from build123d import *

# Parameters (mm, degrees)
SKETCH1_W                   = 42.3
SKETCH1_H                   = 46
SKETCH1_R                   = 12
SKETCH1_R_2                 = 1.7
BOSS_EXTRUDE1_DEPTH         = 2
BOSS_EXTRUDE4_DEPTH         = 2
BOSS_EXTRUDE6_REACH         = 76.681
SKETCH6_W                   = 2
SKETCH6_H                   = 39
M3_TAPPED_HOLE2_D           = 2.5
M3_TAPPED_HOLE2_CSINK_D     = 3.05
M3_TAPPED_HOLE2_CSINK_ANGLE = 90


with BuildPart() as part:
    # Sketch1 → Boss-Extrude1 (new body)
    with BuildSketch(Plane.XY):
        Rectangle(SKETCH1_W, SKETCH1_H)
        Circle(SKETCH1_R, mode=Mode.SUBTRACT)
        with Locations((-15.5, 15.5)):
            Circle(SKETCH1_R_2, mode=Mode.SUBTRACT)
        with Locations((15.5, 15.5)):
            Circle(SKETCH1_R_2, mode=Mode.SUBTRACT)
        with Locations((15.5, -15.5)):
            Circle(SKETCH1_R_2, mode=Mode.SUBTRACT)
        with Locations((-15.5, -15.5)):
            Circle(SKETCH1_R_2, mode=Mode.SUBTRACT)
    extrude(amount=BOSS_EXTRUDE1_DEPTH)

    # Sketch4 → Boss-Extrude4 (add)
    with BuildSketch(Plane.XZ.offset(23)):
        with BuildLine():
            Line((-21.15, 0), (38.85, 0))
            Line((38.85, 0), (38.85, 22))
            ThreePointArc((38.85, 22), (32.992135624, 36.142135624), (18.85, 42))
            Line((18.85, 42), (-21.15, 42))
            Line((-21.15, 42), (-22.15, 42))
            Line((-22.15, 42), (-22.15, 0))
            Line((-22.15, 0), (-21.15, 0))
        make_face()
    extrude(amount=BOSS_EXTRUDE4_DEPTH)

    # Boss-Extrude6: up to this face of the body (flat: up to its plane)
    boss_extrude6_end = Plane(part.part.faces().sort_by_distance((7.447529356, -25, 20.426864787))[0])
    # Sketch6 → Boss-Extrude6 (add, up to the picked face)
    with BuildSketch(Plane(origin=(0, 23, 0), x_dir=(1, 0, 0), z_dir=(0, 1, 0)), mode=Mode.PRIVATE) as boss_extrude6_sk1:
        with Locations((-23.15, -23.5)):
            Rectangle(SKETCH6_W, SKETCH6_H)
    boss_extrude6_tool1 = split(extrude(boss_extrude6_sk1.sketch, amount=-BOSS_EXTRUDE6_REACH, mode=Mode.PRIVATE), bisect_by=boss_extrude6_end, keep=Keep.BOTH, mode=Mode.PRIVATE)
    add(boss_extrude6_tool1.solids().sort_by(Axis((-23.15, 23, 23.5), (0, -1, 0)))[0])

    # M3 Tapped Hole2 (through all)
    with Locations(Plane(origin=(-24.15, 7.5, 12.5), x_dir=(0, 0, -1), z_dir=(-1, 0, 0))):
        with Locations((0, 0), (-20, 0), (-20, 20), (0, 20)):
            CounterSinkHole(M3_TAPPED_HOLE2_D / 2, M3_TAPPED_HOLE2_CSINK_D / 2, counter_sink_angle=M3_TAPPED_HOLE2_CSINK_ANGLE)


solid = part.part
Build history of the part. All positions in model axes, mm. A direction names the side the tool comes from. Coordinates: 2 decimals unless noted, no trailing zeros. Order: outer loops, then holes, each group sorted by start corner. A loop starts at its lowest first (then second) coordinate and runs counter-clockwise, first axis right, second up. Notation, with made-up numbers: (48, 48) -> (52, 48) arc R35 cw to (52, 85) -> close; hole circle Ø8 at (7, 6). An arc over 180 degrees is marked (long way). One line per item, written item: value.
(1) Tool access for faces 4 (the flat face through (-23, -1, 43)), 5 (the flat face through (-1, -24, 42)): list every direction of +Z, -Z, +X, -X, +Y, -Y with a clear straight run to the whole face (end or side of a thin tool).
Checked values:
face 4: +Z, +X, -X, +Y, -Y
face 5: +Z, +X, +Y, -Y
(2) Drop flat-ended pins along their axis: pin 1 Ø2 at (x, y) = (-15.5, 15.5) entering from +Z; pin 2 Ø21 at (x, z) = (11, 23.5) entering from +Y; pin 3 Ø10 at (y, z) = (11.5, 33.5) entering from +X; pin 4 Ø0.6 at (y, z) = (-24.5, 1) entering from -X. Give the stop position or say it passes through.
Checked values:
pin 1: through
pin 2: y = -23
pin 3: x = -22.15
pin 4: x = -22.15
(3) Mould opens along X. For faces 1 (the flat face through (21.15, 0, 1)), 2 (the cylindrical face through (-23, 8.26, 11.51)), 3 (the cylindrical face through (-13.93, -16.15, 0.99)) say: pulls with the +X half, pulls with the -X half, needs draft (parallel to the pull), parting line crosses it, or undercut.
Checked values:
face 1: pulls with the +X half
face 2: needs draft
face 3: undercut
(4) Slice it at B-B, the plane y = 18. List the corners of the cut face in (x, z).
Checked values:
outline: (-24.15, 4) -> (-22.15, 4) -> (-22.15, 43) -> (-24.15, 43) -> close; (-21.15, 0) -> (21.15, 0) -> (21.15, 2) -> (-21.15, 2) -> close
(5) Probe line 1 (Z direction, x = -22.55, y = -12.5); line 2 (Y direction, x = -23, z = 12.5); line 3 (Y direction, x = 15.5, z = 0.9). List the from-to ranges inside material, lowest first. Write a range as [from, to].
Checked values:
line 1: [4, 11.25], [13.75, 31.25], [33.75, 43]
line 2: [-25, -13.75], [-11.25, 6.25], [8.75, 23]
line 3: [-25, -17.2], [-13.8, 13.8], [17.2, 23]
(6) Slice it at A-A, the plane x = -15.5. List the corners of the cut face in (y, z).
Checked values:
outline: (-25, 0) -> (-17.2, 0) -> (-17.2, 2) -> (-23, 2) -> (-23, 42) -> (-25, 42) -> close; (-13.8, 0) -> (13.8, 0) -> (13.8, 2) -> (-13.8, 2) -> close; (17.2, 0) -> (23, 0) -> (23, 2) -> (17.2, 2) -> close
(7) Slice it at C-C, the plane y = 0. List the corners of the cut face in (x, z), plus the area to 3 significant figures.
Checked values:
outline: (-24.15, 4) -> (-22.15, 4) -> (-22.15, 43) -> (-24.15, 43) -> close; (-21.15, 0) -> (-12, 0) -> (-12, 2) -> (-21.15, 2) -> close; (12, 0) -> (21.15, 0) -> (21.15, 2) -> (12, 2) -> close
area: 115 mm2
(8) Slice it at D-D, the plane z = 5. List the corners of the cut face in (x, y).
Checked values:
outline: (-24.15, -25) -> (38.85, -25) -> (38.85, -23) -> (-22.15, -23) -> (-22.15, 23) -> (-24.15, 23) -> close
